Verification items for the finished model (mm, model axes). Coordinates: 2 decimals unless noted, no trailing zeros. Order: outer loops, then holes, each group sorted by start corner. A loop starts at its lowest first (then second) coordinate and runs counter-clockwise, first axis right, second up. Notation, with made-up numbers: M 68,-11 L 106,-11 A18 ccw 106,-6 Z; hole C -8,61.5 d11. An arc over 180 degrees is marked long. Return JSON: item names as keys, results as strings. Group by question number.
Q1. Thickness scan on probe 1 along X at (y, z) = (2.15, -20) (3 decimals); probe 2 along X at (y, z) = (2.45, -5); probe 3 along X at (y, z) = (1, -18). Record the ranges inside material, lowest first.
Q2. Go/stop test with flat-tipped pins: pin 1 Ø5.5 at (x, z) = (-31.675, -20) entering from +Y; pin 2 Ø6 at (x, z) = (-13, -33) entering from -Y. Record where each tip stops, or that it passes through.
Q3. Section check B-B, the plane z = -5. Enter the section's corners in (x, y).
Q4. Section check A-A, the plane x = -5. Enter the section's corners in (y, z), then the cut area to 3 significant figures.
Q5. Section check C-C, the plane y = 2.3. Enter the section's corners in (x, z) (3 decimals), then the cut area to 3 significant figures.
from build123d import *

# Parameters (mm, degrees)
SKETCH1_W           = 110
SKETCH1_H           = 40
SKETCH1_R           = 1.5
BOSS_EXTRUDE1_DEPTH = 3
SKETCH1_6_R         = 3
CUT_EXTRUDE2_DEPTH  = 16


with BuildPart() as part:
    # Sketch1 → Boss-Extrude1 (new body)
    with BuildSketch(Plane(origin=(0, 0, 0), x_dir=(1, 0, 0), z_dir=(0, 1, 0))):
        with Locations((-55, 20)):
            Rectangle(SKETCH1_W, SKETCH1_H)
        with Locations(Location((-95.675, 29, 0), (0, 0, 270))):
            Circle(SKETCH1_R, mode=Mode.SUBTRACT)
        with Locations(Location((-95.675, 11, 0), (0, 0, 270))):
            Circle(SKETCH1_R, mode=Mode.SUBTRACT)
        with Locations(Location((-5, 35, 0), (0, 0, 270))):
            Circle(SKETCH1_R, mode=Mode.SUBTRACT)
        with Locations(Location((-5, 5, 0), (0, 0, 270))):
            Circle(SKETCH1_R, mode=Mode.SUBTRACT)
    extrude(amount=BOSS_EXTRUDE1_DEPTH)

    # Sketch1_6 → Cut-Extrude2 (cut)
    with BuildSketch(Plane(origin=(0, 0, 0), x_dir=(1, 0, 0), z_dir=(0, 1, 0))):
        with Locations(Location((-67.675, 20, 0), (0, 0, 270))):
            Circle(SKETCH1_6_R)
        with Locations(Location((-31.675, 20, 0), (0, 0, 270))):
            Circle(SKETCH1_6_R)
    extrude(amount=CUT_EXTRUDE2_DEPTH, mode=Mode.SUBTRACT)


solid = part.part
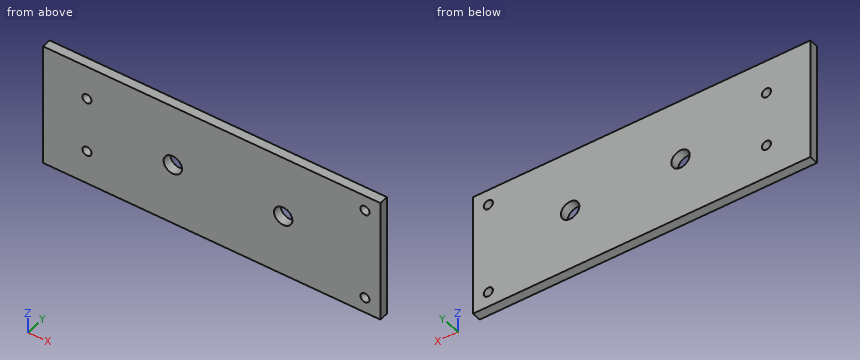
Numbers:
{
 "1": {"probe 1": "x = -110 to -70.675, -64.675 to -34.675, -28.675 to 0", "probe 2": "x = -110 to -6.5, -3.5 to 0", "probe 3": "x = -110 to -69.91, -65.44 to -33.91, -29.44 to 0"},
 "2": {"pin 1": "passes through", "pin 2": "stops at y = 0"},
 "3": {"outline": "M -110,0 L -6.5,0 L -6.5,3 L -110,3 Z; M -3.5,0 L 0,0 L 0,3 L -3.5,3 Z"},
 "4": {"outline": "M 0,-40 L 3,-40 L 3,-36.5 L 0,-36.5 Z; M 0,-33.5 L 3,-33.5 L 3,-6.5 L 0,-6.5 Z; M 0,-3.5 L 3,-3.5 L 3,0 L 0,0 Z", "area": "102 mm2"},
 "5": {"outline": "M -110,-40 L 0,-40 L 0,0 L -110,0 Z; hole C -95.675,-29 d3; hole C -95.675,-11 d3; hole C -67.675,-20 d6; hole C -31.675,-20 d6; hole C -5,-35 d3; hole C -5,-5 d3", "area": "4,320 mm2"}
}
